Could you check a few things on this model? Use its own coordinates, in mm. A direction names the side the tool comes from. Give positions to 0.01 mm unless a question says otherwise; leave off trailing zeros. Order: outer loops, then holes, each group sorted by start corner. A loop starts at its lowest first (then second) coordinate and runs counter-clockwise, first axis right, second up. Notation, with made-up numbers: (1.5, 16.25) -> (53.5, 16.25) arc R5 cw to (53.5, 24.25) -> close; hole circle Ø6 at (64, -11). An arc over 180 degrees is marked (long way). One line per item, written item: value.
```python
from build123d import *

# Parameters (mm, degrees)
SKETCH1_R           = 1.45
BOSS_EXTRUDE1_DEPTH = 5
CUT_EXTRUDE2_DEPTH  = 46.350212776
SKETCH5_W           = 3.6
SKETCH5_H           = 5
FILLET1_R           = 1


with BuildPart() as part:
    # Sketch1 → Boss-Extrude1 (new body)
    with BuildSketch(Plane.XY.offset(1.9)):
        with BuildLine():
            Line((2.45, -8.139256723), (2.45, -4.358612164))
            ThreePointArc((2.45, -4.358612164), (5, 0), (2.45, 4.358612164))
            Line((2.45, 4.358612164), (2.45, 41))
            ThreePointArc((2.45, 41), (0, 43.45), (-2.45, 41))
            Line((-2.45, 41), (-2.45, 8.139256723))
            ThreePointArc((-2.45, 8.139256723), (-2.710254715, 8.056334116), (-2.967710696, 7.965092167))
            Line((-2.967710696, 7.965092167), (-3.054167872, 8.093270203))
            ThreePointArc((-3.054167872, 8.093270203), (-4.342095244, 9.472160372), (-5.994566265, 10.382893341))
            ThreePointArc((-5.994566265, 10.382893341), (-6.032083889, 8.496444973), (-5.481893659, 6.691622066))
            Line((-5.481893659, 6.691622066), (-5.414116812, 6.552658937))
            ThreePointArc((-5.414116812, 6.552658937), (-6.01040764, 6.01040764), (-6.552658937, 5.414116812))
            Line((-6.552658937, 5.414116812), (-6.691622066, 5.481893659))
            ThreePointArc((-6.691622066, 5.481893659), (-8.496444973, 6.032083889), (-10.382893341, 5.994566265))
            ThreePointArc((-10.382893341, 5.994566265), (-9.472160372, 4.342095244), (-8.093270203, 3.054167872))
            Line((-8.093270203, 3.054167872), (-7.965092167, 2.967710696))
            ThreePointArc((-7.965092167, 2.967710696), (-8.210369523, 2.199961883), (-8.381827508, 1.41243323))
            Line((-8.381827508, 1.41243323), (-8.536061531, 1.401648136))
            ThreePointArc((-8.536061531, 1.401648136), (-10.374179133, 0.975715399), (-11.989132531, 0))
            ThreePointArc((-11.989132531, 0), (-10.374179133, -0.975715399), (-8.536061531, -1.401648136))
            Line((-8.536061531, -1.401648136), (-8.381827508, -1.41243323))
            ThreePointArc((-8.381827508, -1.41243323), (-8.210369523, -2.199961883), (-7.965092167, -2.967710696))
            Line((-7.965092167, -2.967710696), (-8.093270203, -3.054167872))
            ThreePointArc((-8.093270203, -3.054167872), (-9.472160372, -4.342095244), (-10.382893341, -5.994566265))
            ThreePointArc((-10.382893341, -5.994566265), (-8.496444973, -6.032083889), (-6.691622066, -5.481893659))
            Line((-6.691622066, -5.481893659), (-6.552658937, -5.414116812))
            ThreePointArc((-6.552658937, -5.414116812), (-6.01040764, -6.01040764), (-5.414116812, -6.552658937))
            Line((-5.414116812, -6.552658937), (-5.481893659, -6.691622066))
            ThreePointArc((-5.481893659, -6.691622066), (-6.032083889, -8.496444973), (-5.994566265, -10.382893341))
            ThreePointArc((-5.994566265, -10.382893341), (-4.342095244, -9.472160372), (-3.054167872, -8.093270203))
            Line((-3.054167872, -8.093270203), (-2.967710696, -7.965092167))
            ThreePointArc((-2.967710696, -7.965092167), (-2.212026244, -8.207127384), (-1.437064557, -8.377639611))
            Line((-1.437064557, -8.377639611), (-1.984198903, -9.839001099))
            Line((-1.984198903, -9.839001099), (-0.052960828, -8.499835007))
            ThreePointArc((-0.052960828, -8.499835007), (1.212003867, -8.413147249), (2.45, -8.139256723))
        make_face()
        with Locations((0, 41)):
            Circle(SKETCH1_R, mode=Mode.SUBTRACT)
    extrude(amount=-BOSS_EXTRUDE1_DEPTH)

    # Sketch4 → Cut-Extrude2 (cut, through all)
    with BuildSketch(Plane.XY.offset(1.9)):
        with BuildLine():
            Line((-5.102940329, -2.6), (-1.358771093, -3.333727811))
            ThreePointArc((-1.358771093, -3.333727811), (-3.6, 0), (-1.358771093, 3.333727811))
            Line((-1.358771093, 3.333727811), (-5.102940329, 2.6))
            Line((-5.102940329, 2.6), (-5.102940329, -2.6))
        make_face()
    extrude(amount=-CUT_EXTRUDE2_DEPTH, mode=Mode.SUBTRACT)

    # Sketch5 → Cut-Revolve1 (revolve, cut)
    with BuildSketch(Plane(origin=(0, 0, 0), x_dir=(1, 0, 0), z_dir=(0, 1, 0))):
        with Locations((1.8, 0.6)):
            Rectangle(SKETCH5_W, SKETCH5_H)
    revolve(axis=Axis((0, 0, -3.1), (0, 0, 1)), mode=Mode.SUBTRACT)

    # Chamfer1
    # the kernel refuses this chamfer: 1.996823512, 1.412365401 mm, written as the material it takes off along each edge
    with BuildSketch(Plane(origin=(-5.994566265, -10.382893341, 6.307600342), x_dir=(0.8971018613244867, 0.44182377754953556, 0), z_dir=(0, 0, -1)), Plane(origin=(-10.382893341, -5.994566265, 6.307600342), x_dir=(0.9978248904640776, -0.06592031530834441, 0), z_dir=(0, 0, -1)), Plane(origin=(-11.989132531, 0, 6.307600342), x_dir=(0.8311815460161395, -0.5560011129145519, 0), z_dir=(0, 0, -1)), Plane(origin=(-10.382893341, 5.994566265, 6.307600342), x_dir=(0.4418237775496057, -0.8971018613244522, 0), z_dir=(0, 0, -1)), Plane(origin=(-5.994566265, 10.382893341, 6.307600342), x_dir=(-0.06592031530837167, -0.9978248904640757, 0), z_dir=(0, 0, -1))) as chamfer1_piece_1:
        with BuildLine():
            Line((1.33889649, 0), (0.700148491, -1.556942978))
            ThreePointArc((0.700148491, -1.556942978), (0.305807457, -0.828670891), (0, 0))
            ThreePointArc((0, 0), (0.684607685, 0.037444556), (1.33889649, 0))
        make_face()
    extrude(amount=13.815200684, mode=Mode.SUBTRACT)

    # Fillet1
    fillet1_edges = [part.edges().sort_by_distance(p)[0] for p in [
        (-1.437064557, -8.377639611, -0.6),
    ]]
    fillet(fillet1_edges, radius=FILLET1_R)


solid = part.part
```
1) If I drill on line 1 along Y through (x, z) = (0, -0.55); line 2 along Y through (x, z) = (0.75, -2); line 3 along X through (y, z) = (23, -2.55), over which ranges is the centre line in solid material (lowest first)?
Answer below:
line 1: y = -8.5 to -3.6, 3.6 to 39.55, 42.45 to 43.45
line 2: y = -8.47 to -3.52, 3.52 to 39.76, 42.24 to 43.33
line 3: x = -2.45 to 2.45
2) Suppose I cut it at A-A, the plane x = 3. Write out the boundary of the cut face in (y, z), then the cut area to 3 significant figures.
Answer below:
outline: (-4, -3.1) -> (-1.99, -3.1) -> (-1.99, 1.9) -> (-4, 1.9) -> close; (1.99, -3.1) -> (4, -3.1) -> (4, 1.9) -> (1.99, 1.9) -> close
area: 20.1 mm2
3) Suppose I cut it at D-D, the plane z = 0.95. State how many separate pieces and enclosed holes the cut face has, then the cut area to 3 significant figures.
Answer below:
separate pieces: 1
enclosed holes: 2
area: 309 mm2
4) Suppose I cut it at C-C, the plane x = 1. Write out the boundary of the cut face in (y, z).
Answer below:
outline: (-8.44, -3.1) -> (-3.46, -3.1) -> (-3.46, 1.9) -> (-8.44, 1.9) -> close; (3.46, -3.1) -> (39.95, -3.1) -> (39.95, 1.9) -> (3.46, 1.9) -> close; (42.05, -3.1) -> (43.24, -3.1) -> (43.24, 1.9) -> (42.05, 1.9) -> close
5) For P1, Ø1.5, axis at y = 28, z = -0.5, coming from the +X side; P2, Ø4.5, axis at x = 0, y = 0, coming from the -Z side; P3, Ø1, axis at x = 0, z = -0.5, coming from the -Y side; P4, Ø1.5, axis at x = -6, z = -2, coming from the -Y side, each with a flat end and sliding along its axis, tell me the tip position at first contact or that it passes through.
Answer below:
P1: stops at x = 2.45
P2: passes through
P3: stops at y = -8.81
P4: stops at y = -9.39
6) For faces 4 (the cylindrical face through (-9.756, -1.188, -0.565)), 5 (the cylindrical face through (-3.849, -9.043, -0.565)), 6 (the flat face through (-10.71, 0.07, -0.57)), 7 (the flat face through (2.45, -6, -1)), 8 (the flat face through (-3.26, -2.96, -0.56)), which set-ups out of +Z, -Z, +X, -X, +Y, -Y let a thin tool reach every point of the face, with its end or its side?
Answer below:
face 4: +Z, -Z, -X
face 5: +Z, -Z, -Y
face 6: +Z, -Z, -X, +Y
face 7: +Z, -Z, +X, -Y
face 8: +Z, -Z
7) We'd pull the mould along Y, two halves only. Please class faces 1 (the cylindrical face through (-7.65, 5.85, -0.56)), 2 (the cylindrical face through (-5.85, -7.65, -0.56)), 3 (the flat face through (-1, 11, 1.9)): +Y half, -Y half, draft (parallel to the pull), parting line (faces both ways), or undercut.
Answer below:
face 1: +Y half
face 2: undercut
face 3: draft
8) Suppose I cut it at B-B, the plane y = 0. Write out the boundary of the cut face in (x, z).
Answer below:
outline: (-10.73, -3.1) -> (-5.1, -3.1) -> (-5.1, 1.9) -> (-10.73, 1.9) -> close; (3.6, -3.1) -> (5, -3.1) -> (5, 1.9) -> (3.6, 1.9) -> close
